Autodesk Inventor part; units mm, degrees
ref_plane "YZ Plane" through (0, 0, 0) normal (1, 0, 0) x (0, 1, 0)
ref_plane "XZ Plane" through (0, 0, 0) normal (0, 1, 0) x (-1, 0, 0)
ref_plane "XY Plane" through (0, 0, 0) normal (0, 0, 1) x (1, 0, 0)
sketch "Sketch1" plane through (0, 0, 0) normal (1, 0, 0) x (0, 1, 0)
  line L0 (0, 0) -> (32.73, 0)
  line L1 (34, 1.27) -> (34, 1.5875)
  line L2 (31.6505, 1.5875) -> (0, 1.5875)
  line L3 (0, 1.5875) -> (0, 0)
  line L4 (34, 6) -> (32.4125, 6)
  line L5 (32.4125, 4.73) -> (32.4125, 2.3495)
  line L6 (33.6825, 6) -> (57.8125, 6)
  line L7 (57.8125, 6) -> (57.8125, 4.4125)
  line L8 (57.8125, 4.4125) -> (34.762, 4.4125)
  arc A0 (34.762, 4.4125) -> (34, 3.6505) centre (34.762, 3.6505) ccw
  arc A1 (31.6505, 1.5875) -> (32.4125, 2.3495) centre (31.6505, 2.3495) ccw
  arc A2 (32.73, 0) -> (34, 1.27) centre (32.73, 1.27) ccw
  arc A3 (33.6825, 6) -> (32.4125, 4.73) centre (33.6825, 4.73) ccw
  line L9 (34, 3.6505) -> (34, 1.5875)
  point P0 (32.4125, 0)
  dimension "d0" = 34
  dimension "d1" = 1.5875
  dimension "d3" = 1.5875
  dimension "d4" = 25.4
  dimension "d5" = 1.5875
  dimension "d7" = 1.27
extrude "Extrusion1" add sketch "Sketch1" along normal blind 59
sketch "Sketch2" plane through (0, 57.8125, 6) normal (0, 1, 0) x (1, 0, 0)
  line L0 (0, 0) -> (59, 0)
  line L1 (0, 1.5875) -> (59, 1.5875)
  line L2 (0, 0) -> (9, 0)
  line L3 (59, 0) -> (50, 0)
  line L4 (50, 0) -> (9, 0)
  line L5 (9, 0) -> (9, 6.35)
  line L6 (9, 6.35) -> (50, 6.35)
  line L7 (50, 6.35) -> (50, 0)
  point P0 (0, 6)
  dimension "d10" = 9
  dimension "d11" = 9
extrude "Extrusion2" cut sketch "Sketch2" against normal blind 28.5
sketch "Sketch3" plane through (0, 0, 1.5875) normal (0, 0, 1) x (1, 0, 0)
  line L0 (50, 29.3125) -> (9, 29.3125)
  circle A0 centre (38.0547, 16) radius 4.0005
  line L1 (48.0547, 8) -> (22.0547, 8)
  line L2 (48.0547, 8) -> (22.0547, 8) construction
  line L3 (48.0547, 9.8542) -> (22.0547, 9.8542)
  line L4 (22.0547, 6.1458) -> (48.0547, 6.1458)
  arc A1 (48.0547, 6.1458) -> (48.0547, 9.8542) centre (48.0547, 8) ccw
  arc A2 (22.0547, 9.8542) -> (22.0547, 6.1458) centre (22.0547, 8) ccw
  line L5 (48.0547, 24) -> (22.0547, 24) construction
  line L6 (48.0547, 22.1458) -> (22.0547, 22.1458)
  line L7 (22.0547, 25.8542) -> (48.0547, 25.8542)
  arc A3 (48.0547, 22.1458) -> (48.0547, 25.8542) centre (48.0547, 24) ccw
  arc A4 (22.0547, 25.8542) -> (22.0547, 22.1458) centre (22.0547, 24) ccw
  line L8 (30.0547, 16) -> (13.0547, 16)
  line L9 (30.0547, 16) -> (13.0547, 16) construction
  line L10 (30.0547, 17.8669) -> (13.0547, 17.8669)
  line L11 (13.0547, 14.1331) -> (30.0547, 14.1331)
  arc A5 (30.0547, 14.1331) -> (30.0547, 17.8669) centre (30.0547, 16) ccw
  arc A6 (13.0547, 17.8669) -> (13.0547, 14.1331) centre (13.0547, 16) ccw
  point P0 (35.0547, 8)
  point P1 (21.5547, 16)
  dimension "d21" = 17
  dimension "d22" = 3.7338
extrude "Extrusion3" cut sketch "Sketch3" against normal blind 28.5
sketch "Sketch4" plane through (0, 33.6825, 6) normal (0, 0, 1) x (1, 0, 0)
  line L0 (50, 24.13) -> (50, 0)
  line L1 (50, 0) -> (59, 0)
  line L2 (59, 24.13) -> (59, 0)
  line L3 (50, 24.13) -> (59, 24.13)
  circle A0 centre (5.4991, 18.13) radius 1.8542
  circle A1 centre (5.4991, 8.1224) radius 1.8542
  circle A2 centre (53.4991, 18.13) radius 1.8542
  circle A3 centre (53.4991, 8.1224) radius 1.8542
  point P0 (0, -33.6825)
extrude "Extrusion4" cut sketch "Sketch4" against normal blind 28.5 contours A0 | A1 | A2 | A3
properties part number "Side Servo Mount"
The listing builds one solid part. Answer for the finished solid, in the listing's coordinates (mm). A direction names the side the tool comes from. Give positions to 0.01 mm unless a question says otherwise; leave off trailing zeros. Order: outer loops, then holes, each group sorted by start corner. A loop starts at its lowest first (then second) coordinate and runs counter-clockwise, first axis right, second up. Notation, with made-up numbers: (88, -9.75) - (110, -9.75) arc R22 ccw to (110, 24.25) - close; hole circle Ø8 at (68.25, -40). An arc over 180 degrees is marked (long way). Answer in a Markdown table with one row per item. Add a question column.
Q1. The part is cut by section D-D (y = 24). Determine the outline of the cut face in (x, z).
Q2. Given P1, Ø2, axis at x = 11.5, y = 6, coming from the +Z side; P2, Ø0.8, axis at x = 20, z = 1, coming from the +Y side; P3, Ø0.7, axis at x = 54, z = 2.5, coming from the +Y side, each flat-ended and moving along its own axis, determine where each tip first touches the part or whether it passes through.
Q3. Find the intervals of material crossed by line 1 along X through (y, z) = (41, 5.7); line 2 along Y through (x, z) = (31.5, 1.45); line 3 along Y through (x, z) = (51.5, 4.7), in increasing order. Write a range as [from, to].
Q4. The part is cut by section C-C (x = 53.5). Determine the outline of the cut face in (y, z), then the cut area to 3 significant figures.
Q5. For a pull along X with two mould halves and no side action, classify faces 1 (the flat face through (9, 43, 5)), 2 (the flat face through (54, 46, 6)), 3 (the flat face through (59, 29, 1)), 4 (the cylindrical face through (31.92, 15.96, 0.8)) as released by +X, released by -X, zero draft, split by the parting line, or undercut.
Q6. The part is cut by section B-B (x = 26). Determine the outline of the cut face in (y, z), then the cut area to 3 significant figures.
Q7. Which of the six approach directions +Z, -Z, +X, -X, +Y, -Y give full straight-line access (tool end or side, diameter ignored) to faces 5 (the flat face through (0, 29, 1)), 6 (the flat face through (21, 14.133, 1)), 7 (the flat face through (50, 43, 5)), 8 (the flat face through (4, 46, 4.412)), 9 (the cylindrical face through (54.437, 32.775, 5.618))?
Q8. The part is cut by section A-A (y = 16). Determine the outline of the cut face in (x, z).
Determined:
| question | item | result |
|---|---|---|
| 1 | outline | (0, 0) - (20.2, 0) - (20.2, 1.59) - (0, 1.59) - close; (49.91, 0) - (59, 0) - (59, 1.59) - (49.91, 1.59) - close |
| 2 | P1 | stops at z = 1.59 |
| 2 | P2 | stops at y = 29.31 |
| 2 | P3 | stops at y = 34 |
| 3 | line 1 | x = [0, 3.83], [7.17, 9], [50, 51.83], [55.17, 59] |
| 3 | line 2 | y = [0, 6.15], [9.85, 14.82], [17.18, 22.15], [25.85, 29.31] |
| 3 | line 3 | y = [32.41, 57.81] |
| 4 | outline | (0, 0) - (32.73, 0) arc R1.27 ccw to (34, 1.27) - (34, 3.65) arc R0.76 cw to (34.76, 4.41) - (39.95, 4.41) - (39.95, 6) - (33.68, 6) arc R1.27 ccw to (32.41, 4.73) - (32.41, 2.35) arc R0.76 cw to (31.65, 1.59) - (0, 1.59) - close; (43.66, 4.41) - (49.96, 4.41) - (49.96, 6) - (43.66, 6) - close; (53.67, 4.41) - (57.81, 4.41) - (57.81, 6) - (53.67, 6) - close |
| 4 | area | 86.6 mm² |
| 5 | face 1 | undercut |
| 5 | face 2 | zero draft |
| 5 | face 3 | released by +X |
| 5 | face 4 | undercut |
| 6 | outline | (0, 0) - (6.15, 0) - (6.15, 1.59) - (0, 1.59) - close; (9.85, 0) - (14.13, 0) - (14.13, 1.59) - (9.85, 1.59) - close; (17.87, 0) - (22.15, 0) - (22.15, 1.59) - (17.87, 1.59) - close; (25.85, 0) - (29.31, 0) - (29.31, 1.59) - (25.85, 1.59) - close |
| 6 | area | 28.8 mm² |
| 7 | face 5 | +Z, -Z, -X, +Y, -Y |
| 7 | face 6 | +Z, -Z |
| 7 | face 7 | +Z, -Z, +Y |
| 7 | face 8 | -Z, +X, -X, +Y |
| 7 | face 9 | +Z, +X, -X, -Y |
| 8 | outline | (0, 0) - (11.19, 0) - (11.19, 1.59) - (0, 1.59) - close; (31.92, 0) - (34.05, 0) - (34.05, 1.59) - (31.92, 1.59) - close; (42.06, 0) - (59, 0) - (59, 1.59) - (42.06, 1.59) - close |
